Model file for the job. Use its own axes, mm. A direction names the side the tool comes from. Round coordinates to 2 decimals unless told otherwise and drop trailing zeros. Order: outer loops, then holes, each group sorted by start corner. A loop starts at its lowest first (then second) coordinate and runs counter-clockwise, first axis right, second up. Notation, with made-up numbers: M 74,1 L 109,1 A15 cw 109,29 Z; hole C 18,-0.75 d2. An arc over 180 degrees is marked long. Return JSON: item names as keys, results as strings. Group by question number.
Item 1: Slice it at A-A on x = 0. Write the cut outline in (y, z), then the cut area to 3 significant figures.
Item 2: Slice it at D-D on z = -251. Write the cut outline in (x, y).
Item 3: Slice it at B-B on z = 12.5. Write the cut outline in (x, y), then the cut area to 3 significant figures.
Item 4: Slice it at C-C on y = -34. Write the cut outline in (x, z).
Item 5: Pin check, flat tips, straight feed: pin 1 Ø6.5 at (x, y) = (-15, 376) entering from +Z; pin 2 Ø11.5 at (x, y) = (26.5, 193.5) entering from +Z; pin 3 Ø8 at (x, z) = (-30.5, 34) entering from -Y; pin 4 Ø10 at (x, z) = (-81.5, -183) entering from -Y. Stop position of each tip, or through.
Item 6: Probe line 1 along Z through (x, y) = (36.5, 201); line 2 along Y through (x, z) = (85, -139); line 3 along Z through (x, y) = (-1, 133). List the from-to ranges inside material, lowest first.
Item 7: Pull direction Z, two halves, no side cores. Call faces 6 (the face through (-70.47, 374.65, 95.71)), 7 (the face through (13, 0, -1)), 8 (the face through (3.815, -31.306, -24.814)): pulls with the +Z half, pulls with the -Z half, needs draft (parallel to the pull), parting line crosses it, or undercut.
Item 8: Which spindle directions (+Z, -Z, +X, -X, +Y, -Y) get a long thin tool onto all of the face, cutting with end or side? Do faces 1 (the face through (95, 291, -152.4)), 2 (the face through (1, 197, -152.4)), 3 (the face through (63.5, 106, 1)), 4 (the face through (-2, 368.3, -2)), 5 (the face through (1, 375, -152.4)). Say none if no direction does.
from build123d import *

# Parameters (mm, degrees)
SKETCH2_W           = 127
SKETCH2_H           = 152.4
BOSS_EXTRUDE2_DEPTH = 215.9
SKETCH3_W           = 228.6
SKETCH3_H           = 355.6
BOSS_EXTRUDE3_DEPTH = 152.4
SKETCH4_R           = 82.55
BOSS_EXTRUDE4_DEPTH = 88.9
CUT_EXTRUDE1_DEPTH  = 484.643280218
SKETCH6_W           = 152.4
SKETCH6_H           = 203.2
BOSS_EXTRUDE5_DEPTH = 152.4
SKETCH7_R           = 12.7
BOSS_EXTRUDE6_DEPTH = 63.5


with BuildPart() as part:
    # Sketch2 → Boss-Extrude2 (new body)
    with BuildSketch(Plane(origin=(0, 0, 0), x_dir=(1, 0, 0), z_dir=(0, 1, 0))):
        Rectangle(SKETCH2_W, SKETCH2_H)
    extrude(amount=BOSS_EXTRUDE2_DEPTH)

    # Sketch3 → Boss-Extrude3 (add)
    with BuildSketch(Plane(origin=(0, 215.9, 0), x_dir=(1, 0, 0), z_dir=(0, 1, 0))):
        with Locations((0, -25.4)):
            Rectangle(SKETCH3_W, SKETCH3_H)
    extrude(amount=BOSS_EXTRUDE3_DEPTH)

    # Sketch4 → Boss-Extrude4 (add)
    with BuildSketch(Plane.ZY.offset(114.3)):
        with Locations((95.25, 292.1)):
            Circle(SKETCH4_R)
    extrude(amount=-BOSS_EXTRUDE4_DEPTH)

    # Sketch5 → Cut-Extrude1 (cut, through all)
    with BuildSketch(Plane.ZY.offset(114.3)):
        Polygon((152.4, 368.3), (203.2, 292.1), (203.2, 368.3), align=None)
        Polygon((203.2, 215.9), (203.2, 241.3), (177.8, 215.9), align=None)
    extrude(amount=-CUT_EXTRUDE1_DEPTH, mode=Mode.SUBTRACT)

    # Sketch6 → Boss-Extrude5 (add)
    with BuildSketch(Plane(origin=(0, 0, -152.4), x_dir=(-1, 0, 0), z_dir=(0, 0, -1))):
        with Locations((0, 279.4)):
            Rectangle(SKETCH6_W, SKETCH6_H)
    extrude(amount=BOSS_EXTRUDE5_DEPTH)

    # Sketch7 → Boss-Extrude6 (add)
    with BuildSketch(Plane.XZ):
        with Locations(Location((0, -12.7, 0), (0, 0, 270))):
            Circle(SKETCH7_R)
    extrude(amount=BOSS_EXTRUDE6_DEPTH)


solid = part.part
Output values:
{
 "1": {"outline": "M -63.5,-25.4 L 0,-25.4 L 0,-76.2 L 215.9,-76.2 L 215.9,-152.4 L 177.8,-152.4 L 177.8,-304.8 L 381,-304.8 L 381,-152.4 L 368.3,-152.4 L 368.3,152.4 L 292.1,203.2 L 241.3,203.2 L 215.9,177.8 L 215.9,76.2 L 0,76.2 L 0,0 L -63.5,0 Z", "area": "117,000 mm²"},
 "2": {"outline": "M -76.2,177.8 L 76.2,177.8 L 76.2,381 L -76.2,381 Z"},
 "3": {"outline": "M -114.3,215.9 L -63.5,215.9 L -63.5,0 L 63.5,0 L 63.5,215.9 L 114.3,215.9 L 114.3,368.3 L -114.3,368.3 Z", "area": "62,300 mm²"},
 "4": {"outline": "C 0,-12.7 d25.4"},
 "5": {"pin 1": "z = -152.4", "pin 2": "z = 76.2", "pin 3": "y = 0", "pin 4": "through"},
 "6": {"line 1": "-304.8 to -152.4, -76.2 to 76.2", "line 2": "215.9 to 368.3", "line 3": "-76.2 to 76.2"},
 "7": {"face 6": "undercut", "face 7": "needs draft", "face 8": "parting line crosses it"},
 "8": {"face 1": "-Z, +X, +Y, -Y", "face 2": "+X, -X, -Y", "face 3": "+Z, +X, -Y", "face 4": "+X, +Y", "face 5": "+X, -X, +Y"}
}
